from build123d import *
from build123d.topology import SkipClean

# Parameters (mm, degrees)
SKETCH_2_R          = 1
CUT_EXTRUDE_1_DEPTH = 50
SKETCH_3_W          = 30
SKETCH_3_H          = 1.543001366
CUT_EXTRUDE_2_DEPTH = 5
FILLET_1_R          = 1


with BuildPart() as part:
    # 草图1 → 旋转1 (revolve)
    with SkipClean():  # the faces are left unmerged after this step: merging them gives an invalid solid
        with BuildSketch(Plane.XY):
            with BuildLine():
                Line((-57.054109227, 42.647640507), (-58.554109227, 42.647640507))
                Line((-58.554109227, 42.647640507), (-58.554109227, 33.247028335))
                ThreePointArc((-58.554109227, 33.247028335), (-56.797365364, 34.258679156), (-56.790595512, 36.285879333))
                ThreePointArc((-56.790595512, 36.285879333), (-56.987108525, 36.764821339), (-57.054109227, 37.278157209))
                Line((-57.054109227, 37.278157209), (-57.054109227, 42.647640507))
            make_face()
            with BuildLine():
                ThreePointArc((-58.554109227, 44.37170043), (-60.291090766, 43.910268372), (-61.570072895, 42.647640507))
                Line((-61.570072895, 42.647640507), (-60.054109227, 42.647640507))
                Line((-60.054109227, 42.647640507), (-58.554109227, 42.647640507))
                Line((-58.554109227, 42.647640507), (-58.554109227, 44.37170043))
            make_face()
            with BuildLine():
                ThreePointArc((-55.53814556, 42.647640507), (-56.817127689, 43.910268372), (-58.554109227, 44.37170043))
                Line((-58.554109227, 44.37170043), (-58.554109227, 42.647640507))
                Line((-58.554109227, 42.647640507), (-57.054109227, 42.647640507))
                Line((-57.054109227, 42.647640507), (-55.53814556, 42.647640507))
            make_face()
        revolve(axis=Axis((-58.554109227, 44.37170043, 0), (0, -1, 0)))
    add(part.part.scale(1), mode=Mode.REPLACE)  # the faces are merged on a copy

    # 草图2 → 切除-拉伸1 (cut)
    with BuildSketch(Plane(origin=(0, 0, 0), x_dir=(1, 0, 0), z_dir=(0, 1, 0))):
        with Locations((-58.554109227, 0)):
            Circle(SKETCH_2_R)
    extrude(amount=CUT_EXTRUDE_1_DEPTH, mode=Mode.SUBTRACT)

    # 草图3 → 切除-拉伸2 (cut, symmetric)
    with BuildSketch(Plane.XY):
        with Locations((-45.847587109, 34.065831969)):
            Rectangle(SKETCH_3_W, SKETCH_3_H)
    extrude(amount=CUT_EXTRUDE_2_DEPTH, both=True, mode=Mode.SUBTRACT)

    # 圆角1
    # the kernel refuses this fillet: 1 mm, written as the material it takes off along each edge
    with BuildSketch(Plane(origin=(-58.554109227, 34.837332652, 0), x_dir=(1, 0, 0), z_dir=(0, 0, 1))) as fillet_1_piece_1:
        with BuildLine():
            CenterArc((0.873089514, 0.991914174), FILLET_1_R, 277.291097339, 111.588468761)
            Line((1.748726343, 1.474884302), (1.836290026, 1.523181315))
            ThreePointArc((1.836290026, 1.523181315), (1.85033803, 1.498160575), (2.080331258, -0.021703426))
            Line((2.080331258, -0.021703426), (1.982714859, -0.1))
            ThreePointArc((1.982714859, -0.1), (1.49135743, -0.1), (1.012691049, -0.099191417))
            Line((1.012691049, -0.099191417), (1, 0))
        make_face()
    revolve(axis=Axis((-58.554109227, 34.837332652, 0), (0, 1, 0)), mode=Mode.SUBTRACT)


solid = part.part
Geometry: final body of the model. Coordinates: model frame, mm. Round coordinates to 2 decimals unless told otherwise and drop trailing zeros. Loops run counter-clockwise (first coordinate to the right, second up) from the corner with the lowest first, then second, coordinate; pieces in that order, holes last. Notation, with made-up numbers: M -5,29 L 2,29 A36 ccw 2,66 Z; hole C -6,-28.5 d8. An arc over 180 degrees is marked long. One line per question, with ' | ' between items.
(1) Pull-direction query (Y, two-part tool) for faces 1 (the cylindrical face through (-59.744, 40, -0.913)), 2 (the cylindrical face through (-57.6, 39.5, -0.3)); classes: +Y half, -Y half, draft (parallel to the pull), parting line (faces both ways), or undercut.
Check result:
face 1: undercut | face 2: draft
(2) Cut plane A-A on y = 41.5. Return the cut outline in (x, z), plus the area to 3 significant figures.
Check result:
outline: C -58.55,0 d3; hole C -58.55,0 d2 | area: 3.93 mm2
(3) Contact query for flat-ended pins moving along their axis: P1, Ø2, axis at x = -57.5, y = 39, coming from the -Z side; P2, Ø1, axis at x = -59.5, z = -2.5, coming from the +Y side; P3, Ø1, axis at x = -60.5, z = -2, coming from the -Y side. Output: stop coordinate, or through.
Check result:
P1: stops at z = -1.5 | P2: stops at y = 43.62 | P3: stops at y = 42.65
(4) Material intervals for line 1 along X through (y, z) = (39.5, 0); line 2 along Z through (x, y) = (-58.5, 38); line 3 along Z through (x, y) = (-59, 36.75), sorted ascending. Write a range as from..to.
Check result:
line 1: x = -60.05..-59.55, -57.55..-57.05 | line 2: z = -1.5..-1, 1..1.5 | line 3: z = -1.51..-0.9, 0.9..1.51
(5) Cut plane B-B on x = -56.5. Return the cut outline in (y, z).
Check result:
outline: M 42.65,-2.21 A2.83 ccw 42.65,2.21 Z
